Build history of the part. All positions in model axes, mm. Face numbers are marked on the shaded views. A direction names the side the tool comes from. Round coordinates to 2 decimals unless told otherwise and drop trailing zeros. Write each loop counter-clockwise with the first axis right and the second up, starting at its lowest first coordinate (ties: lowest second). Pieces come first, ordered by that corner, then holes.
Item 1: Band-saw the part on A-A, the plane y = -11. Write the cut outline in (x, z), then the cut area to 3 significant figures.
Item 2: 3-axis set-ups, long thin cutter, end or side, ignore diameter. For the marked faces 1 and 2: which of +Z, -Z, +X, -X, +Y, -Y reach the whole face in a straight line?
Item 3: Band-saw the part on B-B, the plane x = 43. Write the cut outline in (y, z), then the cut area to 3 significant figures.
Item 4: Wall check: probe 1 along X at (y, z) = (-27, -27.5); probe 2 along X at (y, z) = (1, 10.5); probe 3 along Y at (x, z) = (78, -9.5). Give the ranges that are in metal, low to high.
Item 5: Band-saw the part on C-C, the plane y = -1. Write the cut outline in (x, z), then the cut area to 3 significant figures.
Item 6: Drop flat-ended pins along their axis: pin 1 Ø2.5 at (x, y) = (69, -1.5) entering from -Z; pin 2 Ø12 at (x, z) = (-36.5, -15.5) entering from +Y; pin 3 Ø1.2 at (y, z) = (30.5, 7.5) entering from +X. Give the stop position or say it passes through.
Item 7: Band-saw the part on D-D, the plane x = 74.5. Write the cut outline in (y, z), then the cut area to 3 significant figures.
Item 8: Mould opens along X. For the marked faces 3, 4 and 5 say: +X half, -X half, draft (parallel to the pull), parting line (faces both ways), or undercut.
```python
from build123d import *

# Parameters (mm, degrees)
BOSS_EXTRUDE1_DEPTH = 50
CUT_EXTRUDE3_DEPTH  = 120.604556769
BOSS_EXTRUDE2_DEPTH = 5
CUT_EXTRUDE4_START  = 35
SKETCH4_W           = 100
SKETCH4_H           = 5
CUT_EXTRUDE4_DEPTH  = 52
SKETCH5_W           = 50
SKETCH5_H           = 9
BOSS_EXTRUDE3_DEPTH = 30


with BuildPart() as part:
    # Sketch1 → Boss-Extrude1 (new, symmetric)
    with BuildSketch(Plane.XY):
        Polygon((-45.5, 30), (-45.5, 35), (-55.5, 35), (-55.5, -35), (55.5, -35), (55.5, 35), (45.5, 35), (45.5, 30), (45.5, -30), (-45.5, -30), align=None)
    extrude(amount=BOSS_EXTRUDE1_DEPTH, both=True)

    # Sketch2 → Cut-Extrude3 (cut, through all)
    with BuildSketch(Plane.XY.offset(50)):
        Polygon((-47.5, 25), (-45.5, 25), (-45.5, 30), (-47.5, 30), (-47.5, 31.5), (-52.5, 31.5), (-52.5, 23.5), (-47.5, 23.5), align=None)
        Polygon((47.5, 23.5), (47.5, 25), (45.5, 25), (45.5, 30), (47.5, 30), (47.5, 31.5), (52.5, 31.5), (52.5, 23.5), align=None)
        Polygon((47.5, -20), (45.5, -20), (45.5, -25), (47.5, -25), (47.5, -26.5), (52.5, -26.5), (52.5, -18.5), (47.5, -18.5), align=None)
        Polygon((-47.5, -18.5), (-47.5, -20), (-45.5, -20), (-45.5, -25), (-47.5, -25), (-47.5, -26.5), (-52.5, -26.5), (-52.5, -18.5), align=None)
    extrude(amount=-CUT_EXTRUDE3_DEPTH, mode=Mode.SUBTRACT)

    # Sketch3 → Boss-Extrude2 (add)
    with BuildSketch(Plane.XY.offset(50)):
        Polygon((10.5, 10), (10.5, -30), (45.5, -30), (45.5, -25), (45.5, -20), (45.5, 10), align=None)
        Polygon((-45.5, 35), (-55.5, 35), (-55.5, -35), (55.5, -35), (55.5, 35), (45.5, 35), (45.5, 30), (47.5, 30), (47.5, 31.5), (52.5, 31.5), (52.5, 23.5), (47.5, 23.5), (47.5, 25), (45.5, 25), (45.5, 10), (45.5, -20), (47.5, -20), (47.5, -18.5), (52.5, -18.5), (52.5, -26.5), (47.5, -26.5), (47.5, -25), (45.5, -25), (45.5, -30), (10.5, -30), (-43.5, -30), (-45.5, -30), (-45.5, -25), (-47.5, -25), (-47.5, -26.5), (-52.5, -26.5), (-52.5, -18.5), (-47.5, -18.5), (-47.5, -20), (-45.5, -20), (-45.5, 10), (-45.5, 25), (-47.5, 25), (-47.5, 23.5), (-52.5, 23.5), (-52.5, 31.5), (-47.5, 31.5), (-47.5, 30), (-45.5, 30), align=None)
        Polygon((-43.5, 10), (-45.5, 10), (-45.5, -20), (-45.5, -25), (-45.5, -30), (-43.5, -30), align=None)
        Polygon((47.5, -20), (45.5, -20), (45.5, -25), (47.5, -25), (47.5, -26.5), (52.5, -26.5), (52.5, -18.5), (47.5, -18.5), align=None)
        Polygon((47.5, 30), (45.5, 30), (45.5, 25), (47.5, 25), (47.5, 23.5), (52.5, 23.5), (52.5, 31.5), (47.5, 31.5), align=None)
        Polygon((-45.5, -25), (-45.5, -20), (-47.5, -20), (-47.5, -18.5), (-52.5, -18.5), (-52.5, -26.5), (-47.5, -26.5), (-47.5, -25), align=None)
        Polygon((-45.5, 25), (-45.5, 30), (-47.5, 30), (-47.5, 31.5), (-52.5, 31.5), (-52.5, 23.5), (-47.5, 23.5), (-47.5, 25), align=None)
    extrude(amount=BOSS_EXTRUDE2_DEPTH)

    # Sketch4 → Cut-Extrude4 (cut)
    with BuildSketch(Plane(origin=(0, 0, 0), x_dir=(1, 0, 0), z_dir=(0, 1, 0)).offset(CUT_EXTRUDE4_START)):
        with Locations((0, 41.5)):
            Rectangle(SKETCH4_W, SKETCH4_H)
    extrude(amount=-CUT_EXTRUDE4_DEPTH, mode=Mode.SUBTRACT)

    # Sketch5 → Boss-Extrude3 (add)
    with BuildSketch(Plane(origin=(55.5, 0, 0), x_dir=(0, 0, -1), z_dir=(1, 0, 0))):
        with Locations((-11.097410489, -0.5)):
            Rectangle(SKETCH5_W, SKETCH5_H)
    extrude(amount=BOSS_EXTRUDE3_DEPTH)


solid = part.part
```
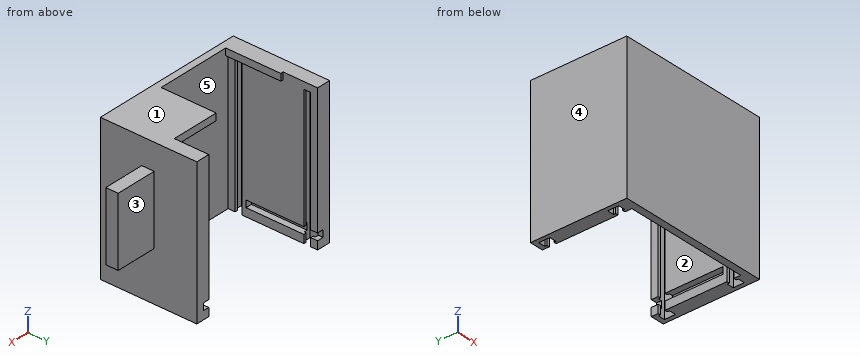
Results:
1. outline: (-55.5, -50) - (-45.5, -50) - (-45.5, -44) - (-50, -44) - (-50, -39) - (-45.5, -39) - (-45.5, 50) - (-43.5, 50) - (-43.5, 55) - (-55.5, 55) - close; (10.5, 50) - (45.5, 50) - (45.5, -39) - (50, -39) - (50, -44) - (45.5, -44) - (45.5, -50) - (55.5, -50) - (55.5, 55) - (10.5, 55) - close
1. area: 2,240 mm2
2. face 1: +Z, +X, -X, +Y, -Y
2. face 2: -Z, +Y
3. outline: (-35, -50) - (-30, -50) - (-30, 50) - (10, 50) - (10, 55) - (-35, 55) - close
3. area: 725 mm2
4. probe 1: x = -55.5 to -45.5, 45.5 to 55.5
4. probe 2: x = -55.5 to -45.5, 45.5 to 85.5
4. probe 3: y = -5 to 4
5. outline: (-55.5, -50) - (-45.5, -50) - (-45.5, -44) - (-50, -44) - (-50, -39) - (-45.5, -39) - (-45.5, 50) - (-43.5, 50) - (-43.5, 55) - (-55.5, 55) - close; (10.5, 50) - (45.5, 50) - (45.5, -39) - (50, -39) - (50, -44) - (45.5, -44) - (45.5, -50) - (55.5, -50) - (55.5, -13.9) - (85.5, -13.9) - (85.5, 36.1) - (55.5, 36.1) - (55.5, 55) - (10.5, 55) - close
5. area: 3,740 mm2
6. pin 1: stops at z = -13.9
6. pin 2: stops at y = -30
6. pin 3: stops at x = 55.5
7. outline: (-5, -13.9) - (4, -13.9) - (4, 36.1) - (-5, 36.1) - close
7. area: 450 mm2
8. face 3: draft
8. face 4: -X half
8. face 5: undercut
